Autodesk Inventor part; units mm, degrees
ref_plane "YZ Plane" through (0, 0, 0) normal (1, 0, 0) x (0, 1, 0)
ref_plane "XZ Plane" through (0, 0, 0) normal (0, 1, 0) x (-1, 0, 0)
ref_plane "XY Plane" through (0, 0, 0) normal (0, 0, 1) x (1, 0, 0)
sketch "Sketch1" plane through (0, 0, 0) normal (0, 1, 0) x (-1, 0, 0)
  line L0 (22.86, 8.89) -> (-22.86, 8.89)
  line L1 (-22.86, 8.89) -> (-22.86, -8.89)
  line L2 (-22.86, -8.89) -> (22.86, -8.89)
  line L3 (22.86, -8.89) -> (22.86, 8.89)
  point P0 (0, 0)
  point P1 (0, -8.89)
  point P2 (22.86, 0)
  dimension "d0" = 45.72
  dimension "d1" = 17.78
extrude "Extrusion1" add sketch "Sketch1" along normal blind 6
sketch "Sketch2" plane through (0, 6, 0) normal (0, 1, 0) x (1, 0, 0)
  line L0 (-7.7772, -6.35) -> (15.5908, -6.35)
  line L1 (15.5908, -6.35) -> (15.5908, 6.35)
  line L2 (15.5908, 6.35) -> (-7.7772, 6.35)
  line L3 (-7.7772, 6.35) -> (-7.7772, -6.35)
  circle A0 centre (-9.86, 0) radius 1.016
  circle A1 centre (17.6736, 0) radius 1.016
  line L4 (-22.86, 8.89) -> (-22.86, -8.89)
  line L5 (22.86, 8.89) -> (-22.86, 8.89)
  point P0 (3.9068, 0)
  point P1 (-7.7772, 0)
  point P2 (3.9068, 6.35)
  dimension "d4" = 23.368
  dimension "d5" = 12.7
  dimension "d6" = 2.032
  dimension "d7" = 2.032
  dimension "d8" = 2.0828
  dimension "d9" = 2.0828
  dimension "d34" = 13
  dimension "d35" = 2.54
extrude "Extrusion2" cut sketch "Sketch2" against normal blind 15
sketch "Sketch3" plane through (22.86, 0, -8.89) normal (0, 0, -1) x (-1, 0, 0)
  line L0 (0, 0) -> (45.72, 0)
  circle A0 centre (22.86, 13.97) radius 3.429
  line L1 (22.86, 17.399) -> (7.9031, 16.12)
  line L2 (22.86, 10.541) -> (7.8514, 10.8324)
  arc A1 (7.9031, 16.12) -> (7.8514, 10.8324) centre (8.1294, 13.4738) ccw
  arc A2 (37.8686, 10.8324) -> (37.8169, 16.12) centre (36.641, 13.4645) ccw
  line L3 (22.86, 17.399) -> (37.8169, 16.12)
  line L4 (22.86, 10.541) -> (37.8686, 10.8324)
  line L5 (45.72, 0) -> (45.72, 6)
  line L6 (45.72, 0) -> (45.72, 7.62)
  line L7 (0, 0) -> (0, 7.62)
  arc A3 (45.72, 7.62) -> (0, 7.62) centre (22.86, 7.62) ccw
  point P0 (22.86, 0)
  point P1 (22.7269, 10.5436)
  point P2 (22.9931, 10.5436)
  point P3 (22.2778, 17.3492)
  point P4 (23.4422, 17.3492)
  point P5 (22.86, 30.48)
  point P6 (39.5451, 13.4929)
  dimension "d14" = 6
  dimension "d15" = 6.858
  dimension "d25" = 7.62
  dimension "d30" = 6
  dimension "d31" = 16.51
  dimension "d33" = 13.781
extrude "Extrusion3" add sketch "Sketch3" along normal blind 3 contours A0 L1 L3 | L2 A1 L1 A0 | A0 L3 A2 L4 | L3 A0
extrude "Extrusion6" add sketch "Sketch3" along normal blind 6 contours L7 A3 L6 L5 L0 | A0 L1 L3 | L2 A1 L1 A0 | A0 L3 A2 L4 | A0 L1 | L3 A0
extrude "Extrusion4" cut sketch "Sketch3" along normal through all contours A0 L1 L3 | A0 L1 | L3 A0
extrude "Extrusion5" cut sketch "Sketch3" along normal blind 3 contours A0 L1 L3 | L2 A1 L1 A0 | A0 L3 A2 L4 | A0 L1 | L3 A0
sketch "Sketch4" plane through (22.86, 0, -8.89) normal (0, 0, 1) x (1, 0, 0)
  line L0 (-22.86, 19.9111) -> (-22.86, 7.8054)
  circle A0 centre (-32.5451, 13.4929) radius 0.75
  circle A1 centre (-36.5451, 13.4929) radius 0.75
  circle A2 centre (-28.5451, 13.4929) radius 0.75
  arc A3 (-37.8169, 16.12) -> (-37.8686, 10.8324) centre (-36.641, 13.4645) ccw
  circle A4 centre (-17.1749, 13.4929) radius 0.75
  circle A5 centre (-13.1749, 13.4929) radius 0.75
  circle A6 centre (-9.1749, 13.4929) radius 0.75
  point P0 (-22.86, 0)
  point P1 (-36.7619, 13.4929)
  point P2 (-39.5451, 13.4929)
  point P3 (-39.5451, 13.4929)
  point P4 (-9.079, 13.4645)
  dimension "d54" = 1.5
  dimension "d55" = 1.5
  dimension "d56" = 1.5
  dimension "d57" = 4
  dimension "d58" = 4
  dimension "d59" = 3
extrude "Extrusion7" cut sketch "Sketch4" against normal blind 4
properties part number "unions1s2"
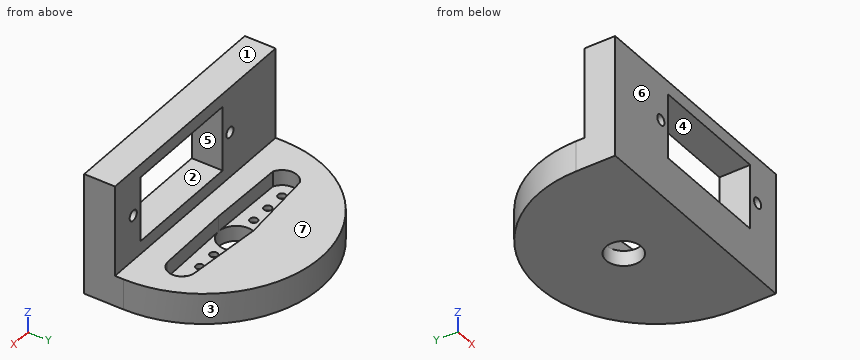
Can you work these out from the model? Positions are in its coordinate system, mm. Face numbers are marked on the shaded views. A direction names the side the tool comes from. Coordinates: 2 decimals unless noted, no trailing zeros. Loops run counter-clockwise (first coordinate to the right, second up) from the corner with the lowest first, then second, coordinate; pieces in that order, holes last. Notation, with made-up numbers: (24, 38.5) - (49, 38.5) arc R9 ccw to (49, 42.5) - close; hole circle Ø7 at (9, 12). An arc over 180 degrees is marked (long way). Use a Markdown table: item, result.
Item 1: For the marked faces 5, 6 and 7, which set-ups out of +Z, -Z, +X, -X, +Y, -Y let a thin tool reach every point of the face, with its end or its side?
Numbers:
| item | result |
|---|---|
| face 5 | +Y, -Y |
| face 6 | +Z, -Z, +X, -X, -Y |
| face 7 | +Z, +X, -X, +Y |
Item 2: I want a section at C-C on x = -9.86. Please give me the cut outline in (y, z), and give its area (3 significant figures).
Numbers:
| item | result |
|---|---|
| outline | (0, -14.89) - (28.24, -14.89) - (28.24, -8.89) - (16.56, -8.89) - (16.56, -11.89) - (14.22, -11.89) - (14.22, -12.89) - (12.76, -12.89) - (12.76, -11.89) - (10.73, -11.89) - (10.73, -8.89) - (6, -8.89) - (6, -1.02) - (0, -1.02) - close; (0, 1.02) - (6, 1.02) - (6, 8.89) - (0, 8.89) - close |
| area | 245 mm2 |
Item 3: We'd pull the mould along X, two halves only. Please class the marked faces 1, 2, 3 and 4: released by +X, released by -X, zero draft, split by the parting line, or undercut.
Numbers:
| item | result |
|---|---|
| face 1 | zero draft |
| face 2 | undercut |
| face 3 | split by the parting line |
| face 4 | undercut |
Item 4: Will these pins go through, and if not, where does the flat tip stop? pin 1 (12 mm diameter, centred on x = 1.5, z = -2.5, fed in from -Y); pin 2 (5 mm diameter, centred on x = -12.5, y = 20.5, fed in from +Z); pin 3 (6 mm diameter, centred on x = 11.5, z = -11, fed in from +Y); pin 4 (1.5 mm diameter, centred on y = 12.5, z = -8.5, fed in from -X).
Numbers:
| item | result |
|---|---|
| pin 1 | stops at y = 0 |
| pin 2 | stops at z = -8.89 |
| pin 3 | stops at y = 28.84 |
| pin 4 | stops at x = -22.46 |
Item 5: If I drill on probe 1 along X at (y, z) = (4.2, 0); probe 2 along X at (y, z) = (2, 3.5); probe 3 along Y at (x, z) = (0, -12.85), over which ranges is the centre line in solid material (lowest first)? Write a range as from..to.
Numbers:
| item | result |
|---|---|
| probe 1 | x = -22.86..-10.88, -8.84..-7.78, 15.59..16.66, 18.69..22.86 |
| probe 2 | x = -22.86..-7.78, 15.59..22.86 |
| probe 3 | y = 0..10.54, 17.4..30.48 |
Item 6: I want a section at A-A on z = 0. Please give me the cut outline in (x, y), and give its area (3 significant figures).
Numbers:
| item | result |
|---|---|
| outline | (-22.86, 0) - (-10.88, 0) - (-10.88, 6) - (-22.86, 6) - close; (-8.84, 0) - (-7.78, 0) - (-7.78, 6) - (-8.84, 6) - close; (15.59, 0) - (16.66, 0) - (16.66, 6) - (15.59, 6) - close; (18.69, 0) - (22.86, 0) - (22.86, 6) - (18.69, 6) - close |
| area | 110 mm2 |
Item 7: I want a section at D-D on y = 7. Please give me the cut outline in (x, z), and give its area (3 significant figures).
Numbers:
| item | result |
|---|---|
| outline | (-22.86, -14.89) - (22.86, -14.89) - (22.86, -8.89) - (-22.86, -8.89) - close |
| area | 274 mm2 |
Item 8: I want a section at B-B on z = -4.5. Please give me the cut outline in (x, y).
Numbers:
| item | result |
|---|---|
| outline | (-22.86, 0) - (-7.78, 0) - (-7.78, 6) - (-22.86, 6) - close; (15.59, 0) - (22.86, 0) - (22.86, 6) - (15.59, 6) - close |
